```python
from build123d import *

# Parameters (mm, degrees)
SKETCH1_W           = 259.398086837
SKETCH1_H           = 83.19083402
BOSS_EXTRUDE1_DEPTH = 3


with BuildPart() as part:
    # Sketch1 → Boss-Extrude1 (new body)
    with BuildSketch(Plane.XY):
        Polygon((816.17673453, 30), (1086.394904374, 30), (1120.574821367, 223.843941842), (1120.574821367, 385), (816.17673453, 385), align=None)
        with Locations((960.875777949, 318.40458299)):
            Rectangle(SKETCH1_W, SKETCH1_H, mode=Mode.SUBTRACT)
    extrude(amount=-BOSS_EXTRUDE1_DEPTH)


solid = part.part
```
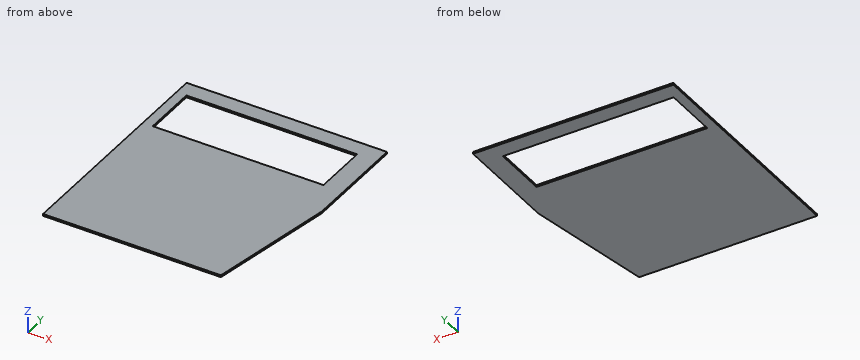
Build history of the part. All positions in model axes, mm. Coordinates: 2 decimals unless noted, no trailing zeros. Write each loop counter-clockwise with the first axis right and the second up, starting at its lowest first coordinate (ties: lowest second). Pieces come first, ordered by that corner, then holes.
1. Drop a flat-ended pin along its axis: pin 1 (3 mm diameter, centred on x = 903.5, y = 171, fed in from +Z). Give the stop position or say it passes through.
Answer block:
pin 1: stops at z = 0
2. Band-saw the part on B-B, the plane z = -1.35. Give the cut face in (x, y).
Answer block:
outline: (816.18, 30) - (1086.39, 30) - (1120.57, 223.84) - (1120.57, 385) - (816.18, 385) - close; hole (831.18, 276.81) - (1090.57, 276.81) - (1090.57, 360) - (831.18, 360) - close
3. Band-saw the part on C-C, the plane y = 307.5. Give the cut face in (x, z).
Answer block:
outline: (816.18, -3) - (831.18, -3) - (831.18, 0) - (816.18, 0) - close; (1090.57, -3) - (1120.57, -3) - (1120.57, 0) - (1090.57, 0) - close
4. Band-saw the part on D-D, the plane y = 191.5. Give the cut face in (x, z).
Answer block:
outline: (816.18, -3) - (1114.87, -3) - (1114.87, 0) - (816.18, 0) - close
5. Drill centre lines: probe 1 along Y at (x, z) = (874.5, -0.4); probe 2 along X at (y, z) = (332.5, -0.15); probe 3 along X at (y, z) = (90.5, -1.15). Where is each one in solid material? Low to high.
Answer block:
probe 1: y = 30 to 276.81, 360 to 385
probe 2: x = 816.18 to 831.18, 1090.57 to 1120.57
probe 3: x = 816.18 to 1097.06
6. Band-saw the part on A-A, the plane x = 946. Give the cut face in (y, z), and give its area (3 significant figures).
Answer block:
outline: (30, -3) - (276.81, -3) - (276.81, 0) - (30, 0) - close; (360, -3) - (385, -3) - (385, 0) - (360, 0) - close
area: 815 mm2
